Geometry check sheet. Reference: the model listing, model coordinates, mm. A direction names the side the tool comes from. Give positions to 0.01 mm unless a question says otherwise; leave off trailing zeros. Loops run counter-clockwise (first coordinate to the right, second up) from the corner with the lowest first, then second, coordinate; pieces in that order, holes last. Notation, with made-up numbers: (77.5, 61.5) -> (105.5, 61.5) arc R14 ccw to (105.5, 66.5) -> close; hole circle Ø5 at (9, 78). An arc over 180 degrees is marked (long way). One line per item, written item: value. Start each with the question number.
(1) Sectioned sample at A-A, the plane x = 6. Record the cut outline in (y, z).
(2) Scan lines: line 1 along Y through (x, z) = (20, -1.45); line 2 along X through (y, z) = (4.75, -5); line 3 along Z through (x, y) = (5.5, -3). Record each from-to range of solid material in increasing order. Write a range as from..to.
(3) Sectioned sample at B-B, the plane x = 20. Record the cut outline in (y, z).
(4) Tool access check on faces 4 (the face through (-7, 0, -2.4)), 5 (the face through (-5, -5, 4.3)), 6 (the face through (17, 0, -10)), 7 (the face through (-6.096, 0.228, 6.518)), 8 (the face through (18, 0, 0)). Record the directions out of +Z, -Z, +X, -X, +Y, -Y that give a thin tool (end or side, any length) a straight path to the whole face; none if there is none.
(5) Draft check along X on faces 1 (the face through (-6, 0, 2)), 2 (the face through (22, 0, -1)), 3 (the face through (21.1, 0, -1.2)). Enter one of: pulls with the +X half, pulls with the -X half, needs draft (parallel to the pull), parting line crosses it, or undercut.
(6) Sectioned sample at C-C, the plane y = -4.5. Record the cut outline in (x, z).
(7) Gauge pin test, flat ends, axial feed: pin 1 Ø2 at (x, y) = (-9, 0) entering from +Z; pin 2 Ø1.5 at (x, y) = (-8, 1) entering from +Z; pin 3 Ø1.5 at (x, y) = (20, 3) entering from -Z; pin 4 Ø6 at (y, z) = (4.5, 8) entering from -X. Record the tip position at first contact, or that the pin passes through.
(8) Sectioned sample at D-D, the plane z = -6.5. Record the cut outline in (x, y), then the cut area to 3 significant figures.
from build123d import *

# Parameters (mm, degrees)
CASE_CONSERVATIVE_PLAN_23X12P2_START     = -18.3
CASE_CONSERVATIVE_PLAN_23X12P2_PROFILE_W = 23
CASE_CONSERVATIVE_PLAN_23X12P2_PROFILE_H = 12.2
CASE_CONSERVATIVE_PLAN_23X12P2_DEPTH     = 22.6
MOUNTING_EARS_33X12P2_START              = -2.4
MOUNTING_EARS_33X12P2_PROFILE_W          = 33
MOUNTING_EARS_33X12P2_PROFILE_H          = 12.2
MOUNTING_EARS_33X12P2_DEPTH              = 2.4
RAISED_GEAR_COVER_ENVELOPE_START         = 4.3
RAISED_GEAR_COVER_ENVELOPE_PROFILE_R     = 6.1
RAISED_GEAR_COVER_ENVELOPE_DEPTH         = 4.5
SECONDARY_GEAR_COVER_ENVELOPE_START      = 4.3
SECONDARY_GEAR_COVER_ENVELOPE_PROFILE_R  = 2.8
SECONDARY_GEAR_COVER_ENVELOPE_DEPTH      = 4.5
OUTPUT_ENVELOPE_NOT_SPLINE_START         = 8.8
OUTPUT_ENVELOPE_NOT_SPLINE_PROFILE_R     = 2.5
OUTPUT_ENVELOPE_NOT_SPLINE_DEPTH         = 3.6
MOUNTING_HOLES_NOMINAL_START             = -50
MOUNTING_HOLES_NOMINAL_PROFILE_R         = 1.1
MOUNTING_HOLES_NOMINAL_DEPTH             = 80.259186592


with BuildPart() as part:
    # Case_conservative_plan_23x12p2_profile → Case_conservative_plan_23x12p2 (new body)
    with BuildSketch(Plane.XY.offset(CASE_CONSERVATIVE_PLAN_23X12P2_START)):
        with Locations((5.5, 0)):
            Rectangle(CASE_CONSERVATIVE_PLAN_23X12P2_PROFILE_W, CASE_CONSERVATIVE_PLAN_23X12P2_PROFILE_H)
    extrude(amount=CASE_CONSERVATIVE_PLAN_23X12P2_DEPTH)

    # Mounting_ears_33x12p2_profile → Mounting_ears_33x12p2 (add)
    with BuildSketch(Plane.XY.offset(MOUNTING_EARS_33X12P2_START)):
        with Locations((5.5, 0)):
            Rectangle(MOUNTING_EARS_33X12P2_PROFILE_W, MOUNTING_EARS_33X12P2_PROFILE_H)
    extrude(amount=MOUNTING_EARS_33X12P2_DEPTH)

    # Raised_gear_cover_envelope_profile → Raised_gear_cover_envelope (add)
    with BuildSketch(Plane.XY.offset(RAISED_GEAR_COVER_ENVELOPE_START)):
        with Locations(Location((0, 0, 0), (0, 0, 169.611142185))):
            Circle(RAISED_GEAR_COVER_ENVELOPE_PROFILE_R)
    extrude(amount=RAISED_GEAR_COVER_ENVELOPE_DEPTH)

    # Secondary_gear_cover_envelope_profile → Secondary_gear_cover_envelope (add)
    with BuildSketch(Plane.XY.offset(SECONDARY_GEAR_COVER_ENVELOPE_START)):
        with Locations((6, 0)):
            Circle(SECONDARY_GEAR_COVER_ENVELOPE_PROFILE_R)
    extrude(amount=SECONDARY_GEAR_COVER_ENVELOPE_DEPTH)

    # Output_envelope_not_spline_profile → Output_envelope_not_spline (add)
    with BuildSketch(Plane.XY.offset(OUTPUT_ENVELOPE_NOT_SPLINE_START)):
        Circle(OUTPUT_ENVELOPE_NOT_SPLINE_PROFILE_R)
    extrude(amount=OUTPUT_ENVELOPE_NOT_SPLINE_DEPTH)

    # Mounting_holes_nominal_profile → Mounting_holes_nominal (cut, through all)
    with BuildSketch(Plane.XY.offset(MOUNTING_HOLES_NOMINAL_START)):
        with Locations(Location((-9, 0, 0), (0, 0, 180))):
            Circle(MOUNTING_HOLES_NOMINAL_PROFILE_R)
        with Locations(Location((20, 0, 0), (0, 0, 180))):
            Circle(MOUNTING_HOLES_NOMINAL_PROFILE_R)
    extrude(amount=MOUNTING_HOLES_NOMINAL_DEPTH, mode=Mode.SUBTRACT)


solid = part.part
Calculated:
1. outline: (-6.1, -18.3) -> (6.1, -18.3) -> (6.1, 4.3) -> (2.8, 4.3) -> (2.8, 8.8) -> (-2.8, 8.8) -> (-2.8, 4.3) -> (-6.1, 4.3) -> close
2. line 1: y = -6.1..-1.1, 1.1..6.1
2. line 2: x = -6..17
2. line 3: z = -18.3..4.3
3. outline: (-6.1, -2.4) -> (-1.1, -2.4) -> (-1.1, 0) -> (-6.1, 0) -> close; (1.1, -2.4) -> (6.1, -2.4) -> (6.1, 0) -> (1.1, 0) -> close
4. face 4: -Z, -X, +Y, -Y
4. face 5: +Z, -X, -Y
4. face 6: -Z, +X, +Y, -Y
4. face 7: +Z
4. face 8: +Z, +X, +Y, -Y
5. face 1: pulls with the -X half
5. face 2: pulls with the +X half
5. face 3: undercut
6. outline: (-11, -2.4) -> (-6, -2.4) -> (-6, -18.3) -> (17, -18.3) -> (17, -2.4) -> (22, -2.4) -> (22, 0) -> (17, 0) -> (17, 4.3) -> (4.12, 4.3) -> (4.12, 8.8) -> (-4.12, 8.8) -> (-4.12, 4.3) -> (-6, 4.3) -> (-6, 0) -> (-11, 0) -> close
7. pin 1: passes through
7. pin 2: stops at z = 0
7. pin 3: stops at z = -2.4
7. pin 4: stops at x = -5.91
8. outline: (-6, -6.1) -> (17, -6.1) -> (17, 6.1) -> (-6, 6.1) -> close
8. area: 281 mm2
